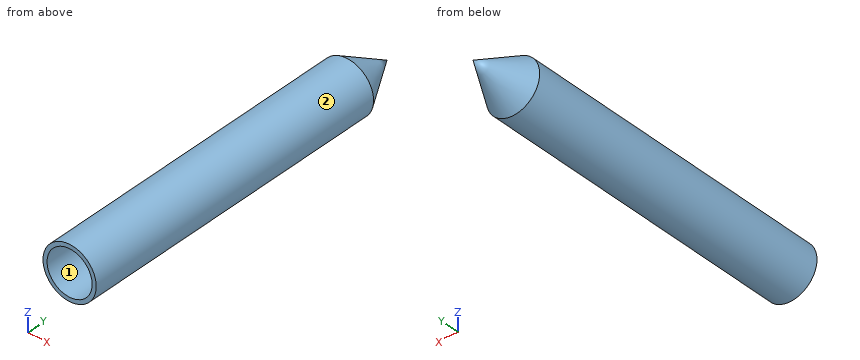
```python
from build123d import *

# Parameters (mm, degrees)
SKETCH1_R           = 15
BOSS_EXTRUDE4_DEPTH = 200
SKETCH1_7_R         = 15
SKETCH1_7_R_2       = 12.7
BOSS_EXTRUDE5_DEPTH = 180


# Read off the part's stored shape, not the designer's step: Draft4
with BuildPart() as part:
    # Sketch1 → Boss-Extrude4 (new body)
    with BuildSketch(Plane(origin=(0, 0, 0), x_dir=(1, 0, 0), z_dir=(0, 1, 0))):
        with Locations(Location((0, 0, 0), (0, 0, 270))):
            Circle(SKETCH1_R)
    extrude(amount=BOSS_EXTRUDE4_DEPTH)

    # Draft4 outline → Draft4 (revolve, cut)
    with BuildSketch(Plane.XY):
        Polygon((15, 0), (15, 200), (0, 200), (0, 25.980762114), align=None)
    revolve(axis=Axis((0, 0, 0), (0, 1, 0)), mode=Mode.SUBTRACT)

    # Sketch1<7> → Boss-Extrude5 (add)
    with BuildSketch(Plane(origin=(0, 0, 0), x_dir=(1, 0, 0), z_dir=(0, 1, 0))):
        with Locations(Location((0, 0, 0), (0, 0, 270))):
            Circle(SKETCH1_7_R)
        with Locations(Location((0, 0, 0), (0, 0, 270))):
            Circle(SKETCH1_7_R_2, mode=Mode.SUBTRACT)
    extrude(amount=-BOSS_EXTRUDE5_DEPTH)


solid = part.part
```
Could you check a few things on this model? Use its own coordinates, in mm. Face numbers are marked on the shaded views. Give positions to 0.01 mm unless a question says otherwise; leave off trailing zeros. Write each loop counter-clockwise with the first axis right and the second up, starting at its lowest first coordinate (ties: lowest second). Pieces come first, ordered by that corner, then holes. Notation, with made-up numbers: (23, -1) - (57, -1) arc R20 cw to (57, 14) - close; hole circle Ø11 at (54, 29). An arc over 180 degrees is marked (long way). One line per item, written item: value. Start each with the question number.
Item 1: Imagine slicing it at A-A, the plane y = -131. List the corners of the cut face in (x, z) for me, and give its area (3 significant figures).
Item 2: If we mould it in two halves opening along Z, with no side actions, what happens to the marked faces 1 and 2? For each: +Z half, -Z half, draft (parallel to the pull), parting line (faces both ways), or undercut.
Item 3: I'm going to push flat-ended pins straight in: pin 1 (4 mm diameter, centred on x = -3, y = -51, fed in from -Z); pin 2 (2 mm diameter, centred on x = -3, y = -129.5, fed in from +Z); pin 3 (10 mm diameter, centred on x = 9.5, z = 9.5, fed in from +Y). Where does each tip first touch, or does it pass through?
Item 4: Please list where these lines run through material, in increasing order: line 1 (X direction, y = -76.5, z = 0); line 2 (X direction, y = -34, z = -11.5); line 3 (Z direction, x = -4.5, y = -26). Write a range as from..to.
Geometry says:
1. outline: circle Ø30 at (0, 0); hole circle Ø25.4 at (0, 0)
1. area: 200 mm^2
2. face 1: undercut
2. face 2: parting line
3. pin 1: z = -14.97
3. pin 2: z = 14.87
3. pin 3: y = 11.37
4. line 1: -15..-12.7, 12.7..15
4. line 2: -9.63..-5.39, 5.39..9.63
4. line 3: -14.31..-11.88, 11.88..14.31
